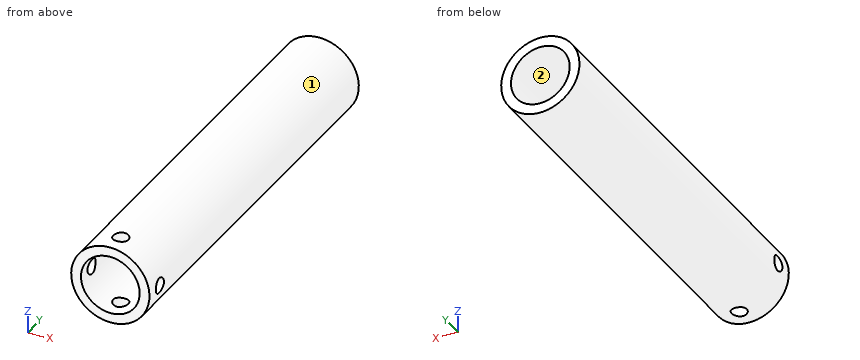
```python
from build123d import *

# Parameters (mm, degrees)
SKETCH1_R          = 12.7
SKETCH1_R_2        = 9.525
ELTUBO_DEPTH       = 127
SETSCREW_OUTLINE_W = 2.45745
SETSCREW_OUTLINE_H = 3.497687322
CIRPATTERN1_COUNT  = 4


# Read off the part's stored shape, not the designer's step: SetScrew
with BuildPart() as part:
    # Sketch1 → ElTubo (new body)
    with BuildSketch(Plane(origin=(0, 0, 0), x_dir=(1, 0, 0), z_dir=(0, 1, 0))):
        with Locations(Location((0, 0, 0), (0, 0, 270))):
            Circle(SKETCH1_R)
        with Locations(Location((0, 0, 0), (0, 0, 270))):
            Circle(SKETCH1_R_2, mode=Mode.SUBTRACT)
    extrude(amount=ELTUBO_DEPTH)

    # SetScrew outline → SetScrew (revolve, cut)
    with BuildSketch(Plane(origin=(0, 6.35, 0), x_dir=(0, 1, 0), z_dir=(0, 0, -1))):
        with Locations((1.228725, -10.951191646)):
            Rectangle(SETSCREW_OUTLINE_W, SETSCREW_OUTLINE_H)
    setscrew = revolve(axis=Axis((0, 6.35, 0), (1, 0, 0)), mode=Mode.SUBTRACT)

    # CirPattern1: SetScrew ×4 about axis
    cirpattern1_axis = Axis((0, 127, 0), (0, -1, 0))
    for i in range(1, CIRPATTERN1_COUNT):
        add(setscrew.rotate(cirpattern1_axis, i * 360 / CIRPATTERN1_COUNT), mode=Mode.SUBTRACT)


solid = part.part
```
Input: part model. Units: mm. Frame: model coordinates. Face numbers are marked on the shaded views. Coordinates: 2 decimals unless noted, no trailing zeros. Loops run counter-clockwise (first coordinate to the right, second up) from the corner with the lowest first, then second, coordinate; pieces in that order, holes last. Notation, with made-up numbers: (75, -29) - (124, -29) arc R6 ccw to (124, -23) - close; hole circle Ø2 at (31, 83). An arc over 180 degrees is marked (long way). Answer in a Markdown table with one row per item.
(1) Mould query, pull axis X, two halves, no side actions, for the marked faces 1 and 2. Classes: pulls with the +X half, pulls with the -X half, needs draft (parallel to the pull), parting line crosses it, or undercut.
Model answer:
| item | result |
|---|---|
| face 1 | parting line crosses it |
| face 2 | undercut |
(2) Cut plane D-D on z = 7.5. Output: boundary loops of the cut face in (x, y), plus the area to 3 significant figures.
Model answer:
| item | result |
|---|---|
| outline | (-10.25, 0) - (-5.87, 0) - (-5.87, 127) - (-10.25, 127) - close; (5.87, 0) - (10.25, 0) - (10.25, 127) - (5.87, 127) - close |
| area | 1,110 mm² |
(3) Pin query (flat end, axial travel): P1, Ø10, axis at x = 9.5, y = 87, coming from the -Z side; P2, Ø3, axis at y = 41.5, z = -2, coming from the -X side; P3, Ø5, axis at x = -3, y = 76, coming from the -Z side. Return the tip coordinate at first contact, or that it passes through.
Model answer:
| item | result |
|---|---|
| P1 | stops at z = -11.88 |
| P2 | stops at x = -12.69 |
| P3 | stops at z = -12.69 |
(4) Cut plane C-C on x = 7.75. Output: boundary loops of the cut face in (y, z), plus the area to 3 significant figures.
Model answer:
| item | result |
|---|---|
| outline | (0, -10.06) - (127, -10.06) - (127, -5.54) - (0, -5.54) - close; (0, 5.54) - (127, 5.54) - (127, 10.06) - (0, 10.06) - close |
| area | 1,150 mm² |
(5) Cut plane A-A on y = 6.35. Output: boundary loops of the cut face in (x, z) (3 decimals), plus the area to 3 significant figures.
Model answer:
| item | result |
|---|---|
| outline | (-12.46, -2.457) arc R12.7 ccw to (-2.457, -12.46) - (-2.457, -9.203) arc R9.525 cw to (-9.203, -2.457) - close; (-12.46, 2.457) - (-9.203, 2.457) arc R9.525 cw to (-2.457, 9.203) - (-2.457, 12.46) arc R12.7 ccw to start; (2.457, -12.46) arc R12.7 ccw to (12.46, -2.457) - (9.203, -2.457) arc R9.525 cw to (2.457, -9.203) - close; (2.457, 9.203) arc R9.525 cw to (9.203, 2.457) - (12.46, 2.457) arc R12.7 ccw to (2.457, 12.46) - close |
| area | 159 mm² |
(6) Material intervals for L1, parallel to Y at x = 10.9, z = 0; L2, parallel to Z at x = -0.5, y = 70.5; L3, parallel to X at y = 75.5, z = 0 (3 decimals), sorted ascending. Write a range as from..to.
Model answer:
| item | result |
|---|---|
| L1 | y = 0..3.89, 8.81..127 |
| L2 | z = -12.69..-9.51, 9.51..12.69 |
| L3 | x = -12.7..-9.525, 9.525..12.7 |
(7) Cut plane B-B on z = 0. Output: boundary loops of the cut face in (x, y) (3 decimals).
Model answer:
| item | result |
|---|---|
| outline | (-12.7, 0) - (-9.525, 0) - (-9.525, 3.893) - (-12.7, 3.893) - close; (-12.7, 8.807) - (-9.525, 8.807) - (-9.525, 127) - (-12.7, 127) - close; (9.525, 0) - (12.7, 0) - (12.7, 3.893) - (9.525, 3.893) - close; (9.525, 8.807) - (12.7, 8.807) - (12.7, 127) - (9.525, 127) - close |
